```python
from build123d import *

# Parameters (mm, degrees)
SKETCH_2_R               = 2.8
EXTRUDE_1_DEPTH          = 120
SKETCH_3_W               = 5.6
SKETCH_3_H               = 1.5
CUT_EXTRUDE_2_DEPTH      = 3.8
CUT_EXTRUDE_6_DEPTH      = 3.8
CUT_EXTRUDE_6_DEPTH_BACK = 0.0001
SCALE_1_SCALE            = 10


with BuildPart() as part:
    # Эскиз2 → Вытянуть1 (new body)
    with BuildSketch(Plane(origin=(0, 0, 0), x_dir=(1, 0, 0), z_dir=(0, 1, 0))):
        Circle(SKETCH_2_R)
    extrude(amount=EXTRUDE_1_DEPTH)

    # Эскиз3 → Вытянуть2 (cut, through all)
    with BuildSketch(Plane.XY):
        with Locations((0, 0.75)):
            Rectangle(SKETCH_3_W, SKETCH_3_H)
    extrude(amount=-CUT_EXTRUDE_2_DEPTH, mode=Mode.SUBTRACT)

    # Эскиз5 → Вырез-Повернуть1 (revolve, cut)
    with BuildSketch(Plane.XY):
        Polygon((-2.375975952, 5.731640408), (-2.8, 5.99660004), (-2.8, 3.466680776), (-2.375975952, 3.731640408), align=None)
    revolve(axis=Axis((0, 0, 0), (0, 1, 0)), mode=Mode.SUBTRACT)

    # Эскиз6 → Вытянуть6 (cut, two sides)
    with BuildSketch(Plane.XY) as cut_extrude_6_sk:
        with BuildLine():
            Line((-2.337778294, 120.351251099), (-2.337778294, 116.645068544))
            ThreePointArc((-2.337778294, 116.645068544), (-2.207612569, 116.330820685), (-1.89336471, 116.20065496))
            Line((-1.89336471, 116.20065496), (1.89336471, 116.20065496))
            ThreePointArc((1.89336471, 116.20065496), (2.207612569, 116.330820685), (2.337778294, 116.645068544))
            Line((2.337778294, 116.645068544), (2.337778294, 120.351251099))
            Line((2.337778294, 120.351251099), (-2.337778294, 120.351251099))
        make_face()
    extrude(amount=CUT_EXTRUDE_6_DEPTH, mode=Mode.SUBTRACT)
    extrude(cut_extrude_6_sk.sketch, amount=-CUT_EXTRUDE_6_DEPTH_BACK, mode=Mode.SUBTRACT)


with BuildPart() as part_1:
    # Масштаб1: scaled about (-2e-09, 59.813507697, -0.010902497)
    add(part.part.scale(SCALE_1_SCALE).moved(Location((1.8e-08, -538.321569273, 0.098122473))))


solid = part_1.part
```
The model under review builds one solid part; all positions refer to its coordinate system, in mm. A direction names the side the tool comes from. Give positions to 0.01 mm unless a question says otherwise; leave off trailing zeros. Write each loop counter-clockwise with the first axis right and the second up, starting at its lowest first coordinate (ties: lowest second). Pieces come first, ordered by that corner, then holes. Notation, with made-up numbers: (14.25, 30.5) -> (56.25, 30.5) arc R27 cw to (56.25, 50.5) -> close; hole circle Ø5 at (20, -4.5). An arc over 180 degrees is marked (long way). Answer in a Markdown table with one row per item.
1) Mouldability with a two-part tool opening along X and no side actions: class faces 4 (the cylindrical face through (26.707, 83.681, -8.312)), 5 (the flat face through (0, 643, 0.097)), 6 (the flat face through (0, -523.322, -11)) as +X half, -X half, draft (parallel to the pull), parting line (faces both ways), or undercut.
Worked answers:
| item | result |
|---|---|
| face 4 | parting line |
| face 5 | undercut |
| face 6 | draft |
2) Tool access review of faces 1 (the conical face through (5.195, -501.134, -23.298)), 2 (the flat face through (0, 623.685, 14)), 3 (the flat face through (0, -538.322, 11)): name each direction out of +Z, -Z, +X, -X, +Y, -Y from which nothing blocks a thin tool from reaching the whole face with its end or side.
Worked answers:
| item | result |
|---|---|
| face 1 | none |
| face 2 | +Z, +Y |
| face 3 | +Z, -Z, +X, -X, -Y |
3) Clearance check with flat-ended pins moving along their axes: P1, Ø1, axis at y = -239, z = 13.5, coming from the +X side; P2, Ø1.5, axis at y = -161.5, z = -12, coming from the -X side; P3, Ø7.5, axis at x = -1, y = -532.5, coming from the -Z side; P4, Ø2, axis at x = -20.5, z = -22, coming from the -Y side. State where each tip first meets the part, or that it passes through.
Worked answers:
| item | result |
|---|---|
| P1 | x = 24.85 |
| P2 | x = -25.6 |
| P3 | z = 0.1 |
| P4 | through |
4) Add section B-B on y = 452. State the section outline as (x, z) points, plus the area to 3 significant figures.
Worked answers:
| item | result |
|---|---|
| outline | circle Ø56 at (0, 0.1) |
| area | 2,460 mm² |
5) Add section A-A on x = 0. State the section outline as (y, z) points, plus the area to 3 significant figures.
Worked answers:
| item | result |
|---|---|
| outline | (-538.32, 0.1) -> (-523.32, 0.1) -> (-523.32, -27.9) -> (-503.65, -27.9) -> (-501.01, -23.66) -> (-481.01, -23.66) -> (-478.36, -27.9) -> (661.68, -27.9) -> (661.68, 0.1) -> (623.68, 0.1) -> (623.68, 28.1) -> (-478.36, 28.1) -> (-481.01, 23.86) -> (-501.01, 23.86) -> (-503.65, 28.1) -> (-538.32, 28.1) -> close |
| area | 65,500 mm² |
6) For L1, parallel to X at y = 409, z = 2.5; L2, parallel to Y at x = -14.5, z = -12.5; L3, parallel to Z at x = -15, y = -455.5, list the stretches that pass through material, from the lowest coordinate up. Write a range as [from, to].
Worked answers:
| item | result |
|---|---|
| L1 | [-27.9, 27.9] |
| L2 | [-523.32, 661.68] |
| L3 | [-23.55, 23.74] |
